```python
from build123d import *

# Parameters (mm, degrees)
SKETCH_2_W          = 2
SKETCH_2_H          = 6.5
CUT_EXTRUDE_1_DEPTH = 10
SKETCH_3_W          = 5.751946122
SKETCH_3_H          = 18.448834599
CUT_EXTRUDE_2_DEPTH = 17.5
SKETCH_4_W          = 3
SKETCH_4_H          = 0.75
EXTRUDE_944_DEPTH   = 5
SKETCH_5_R          = 1
EXTRUDE_1_DEPTH     = 4


with BuildPart() as part:
    # 草图1 → 旋转1 (revolve)
    with BuildSketch(Plane.XY, mode=Mode.PRIVATE) as revolve_1_sk:
        Polygon((0, 0), (0, 5), (2, 7.5), (3, 7.5), (3, 6), (19.5, 6), (19.5, 4), (20.5, 4), (20.5, 0), align=None)
    revolve(revolve_1_sk.sketch.rotate(Axis((0, 0, 0), (1, 0, 0)), 90), axis=Axis((0, 0, 0), (1, 0, 0)))

    # 草图2 → 切除-拉伸1 (cut)
    with BuildSketch(Plane(origin=(0, 0, 0), x_dir=(0, 0, -1), z_dir=(1, 0, 0))):
        Rectangle(SKETCH_2_W, SKETCH_2_H)
    extrude(amount=CUT_EXTRUDE_1_DEPTH, mode=Mode.SUBTRACT)

    # 草图3 → 切除-拉伸2 (cut)
    with BuildSketch(Plane(origin=(20.5, 0, 0), x_dir=(0, 0, -1), z_dir=(1, 0, 0))):
        with Locations((-8.125973061, 0.639105125)):
            Rectangle(SKETCH_3_W, SKETCH_3_H)
        with Locations((8.125973061, 0.639105125)):
            Rectangle(SKETCH_3_W, SKETCH_3_H)
    extrude(amount=-CUT_EXTRUDE_2_DEPTH, mode=Mode.SUBTRACT)

    # 草图4 → Extrude 944 (add)
    with BuildSketch(Plane(origin=(20.5, 0, 0), x_dir=(0, 0, -1), z_dir=(1, 0, 0))):
        with Locations((0, 2.915)):
            Rectangle(SKETCH_4_W, SKETCH_4_H)
        with Locations((0, -2.915)):
            Rectangle(SKETCH_4_W, SKETCH_4_H)
    extrude(amount=EXTRUDE_944_DEPTH)

    # 草图5 → 凸台-拉伸1 (add)
    with BuildSketch(Plane(origin=(20.5, 0, 0), x_dir=(0, 0, -1), z_dir=(1, 0, 0))):
        with Locations(Location((-2.5, 0, 0), (0, 0, 180))):
            Circle(SKETCH_5_R)
        with Locations(Location((2.5, 0, 0), (0, 0, 180))):
            Circle(SKETCH_5_R)
    extrude(amount=EXTRUDE_1_DEPTH)


solid = part.part
```
Part model, mm, in its own coordinate system. A direction names the side the tool comes from. Give positions to 0.01 mm unless a question says otherwise; leave off trailing zeros. Loops run counter-clockwise (first coordinate to the right, second up) from the corner with the lowest first, then second, coordinate; pieces in that order, holes last. Notation, with made-up numbers: M -32.5,39.25 L -15.5,39.25 A8 cw -15.5,47.25 Z; hole C 27.25,38 d4. An arc over 180 degrees is marked long. Return JSON: item names as keys, results as strings.
1) Drill centre lines: line 1 (Z direction, x = 9.75, y = 0); line 2 (Y direction, x = 21.5, z = 1.25). Where is each one in solid material? Low to high.
Calculated:
{"line 1": "z = -5.25 to -1, 1 to 5.25", "line 2": "y = -3.29 to -2.54, 2.54 to 3.29"}
2) Saw through at D-D, the plane x = 22.5. List the corners of the cut face in (y, z).
Calculated:
{"outline": "M -3.29,-1.5 L -2.54,-1.5 L -2.54,1.5 L -3.29,1.5 Z; C 0,-2.5 d2; C 0,2.5 d2; M 2.54,-1.5 L 3.29,-1.5 L 3.29,1.5 L 2.54,1.5 Z"}
3) Saw through at A-A, the plane z = 0. List the corners of the cut face in (x, y), then the cut area to 4 significant figures.
Calculated:
{"outline": "M 0,-5 L 2,-7.5 L 3,-7.5 L 3,-6 L 19.5,-6 L 19.5,-4 L 20.5,-4 L 20.5,-3.29 L 25.5,-3.29 L 25.5,-2.54 L 20.5,-2.54 L 20.5,2.54 L 25.5,2.54 L 25.5,3.29 L 20.5,3.29 L 20.5,4 L 19.5,4 L 19.5,6 L 3,6 L 3,7.5 L 2,7.5 L 0,5 L 0,3.25 L 10,3.25 L 10,-3.25 L 0,-3.25 Z", "area": "188.5 mm2"}
4) Flat gauge pins, fed straight in: pin 1 Ø0.8 at (x, y) = (23, 3) entering from +Z; pin 2 Ø0.9 at (x, z) = (24, 0.5) entering from +Y; pin 3 Ø6.5 at (x, y) = (9, 0) entering from +Z. Where does each tip first touch, or does it go through?
Calculated:
{"pin 1": "stops at z = 1.5", "pin 2": "stops at y = 3.29", "pin 3": "stops at z = 5.25"}
5) Saw through at C-C, the plane y = 0. List the corners of the cut face in (x, z), then the cut area to 3 significant figures.
Calculated:
{"outline": "M 0,-5 L 2,-7.5 L 3,-7.5 L 3,-5.25 L 19.5,-5.25 L 19.5,-4 L 20.5,-4 L 20.5,-3.5 L 24.5,-3.5 L 24.5,-1.5 L 20.5,-1.5 L 20.5,1.5 L 24.5,1.5 L 24.5,3.5 L 20.5,3.5 L 20.5,4 L 19.5,4 L 19.5,5.25 L 3,5.25 L 3,7.5 L 2,7.5 L 0,5 L 0,1 L 10,1 L 10,-1 L 0,-1 Z", "area": "217 mm2"}
6) 3-axis set-ups, long thin cutter, end or side, ignore diameter. For faces 1 (the face through (19.5, -4.1, -1.2)), 2 (the face through (5, 0, 1)), 3 (the face through (23, -3.29, 0)): which of +Z, -Z, +X, -X, +Y, -Y reach the whole face in a straight line?
Calculated:
{"face 1": "+X", "face 2": "-X", "face 3": "+Z, -Z, +X, -Y"}
7) Saw through at B-B, the plane x = 4. List the corners of the cut face in (y, z), then the cut area to 3 significant figures.
Calculated:
{"outline": "M -2.9,-5.25 L 2.9,-5.25 A6 ccw 2.9,5.25 L -2.9,5.25 A6 ccw Z; hole M -3.25,-1 L 3.25,-1 L 3.25,1 L -3.25,1 Z", "area": "94.2 mm2"}
8) Pull direction Z, two halves, no side cores. Call faces 4 (the face through (11, 0, 5.25)), 5 (the face through (5, 3.25, 0)), 6 (the face through (11, -6, 0)), 7 (the face through (0, -0.1, 1.2)): released by +Z, released by -Z, zero draft, split by the parting line, or undercut.
Calculated:
{"face 4": "released by +Z", "face 5": "undercut", "face 6": "split by the parting line", "face 7": "zero draft"}
